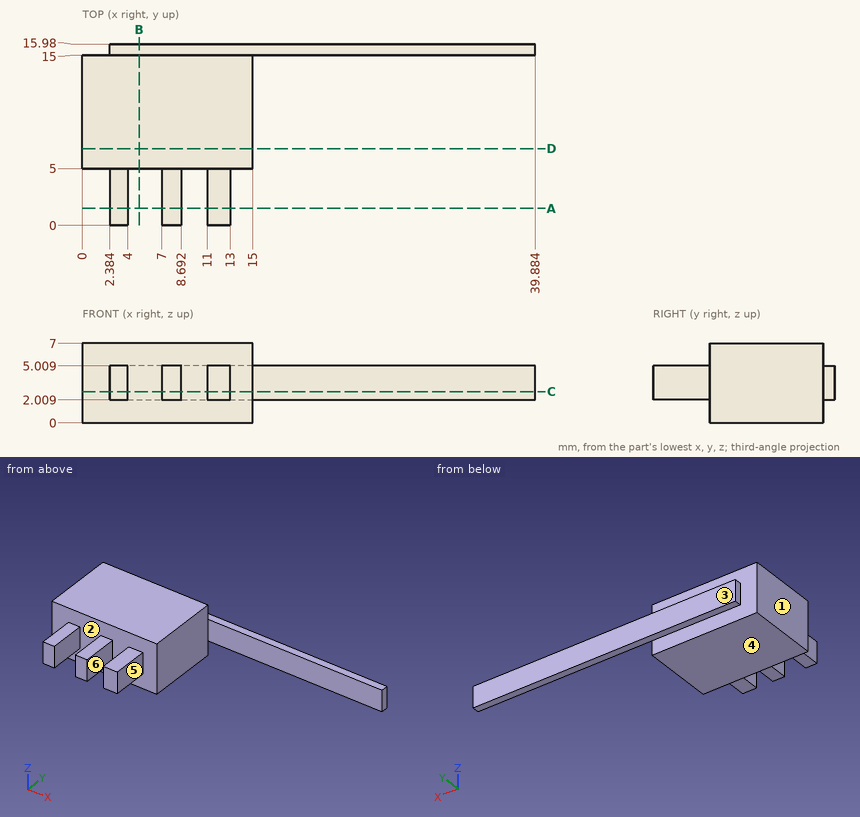
Print and shaded views of the part. All mm, measured from the part's lowest x, y and z. A direction names the side the tool comes from. Give positions to 0.01 mm unless a question says otherwise; leave off trailing zeros. Loops run counter-clockwise (first coordinate to the right, second up) from the corner with the lowest first, then second, coordinate; pieces in that order, holes last. Notation, with made-up numbers: (71.25, 87.5) - (89.25, 87.5) arc R15 cw to (89.25, 115.5) - close; hole circle Ø10 at (-26.5, 7.25). An arc over 180 degrees is marked (long way). One line per item, written item: value. Start each with the question number.
1. Slice it at B-B (x = 5). List the corners of the cut face in (y, z).
2. Pull direction X, two halves, no side cores. Call the marked faces 1, 2 and 3: pulls with the +X half, pulls with the -X half, needs draft (parallel to the pull), parting line crosses it, or undercut.
3. Slice it at A-A (y = 1.5). List the corners of the cut face in (x, z).
4. Slice it at C-C (z = 2.75). List the corners of the cut face in (x, y), plus the area to 3 significant figures.
5. Slice it at D-D (y = 6.75). List the corners of the cut face in (x, z), plus the area to 3 significant figures.
6. Probe L1, parallel to X at y = 12, z = 4.25; L2, parallel to Y at x = 10, z = 4; L3, parallel to Y at x = 14.5, z = 1.75. List the from-to ranges inside material, lowest first. Write a range as from..to.
7. Which spindle directions (+Z, -Z, +X, -X, +Y, -Y) get a long thin tool onto all of the face, cutting with end or side? Do the marked faces 4, 5 and 6. Say none if no direction does.
8. Pin check, flat tips, straight feed: pin 1 (2 mm diameter, centred on x = 12, y = 3, fed in from -Z); pin 2 (0.9 mm diameter, centred on y = 3, z = 3, fed in from +X); pin 3 (1.8 mm diameter, centred on x = 3, y = 2.5, fed in from +Z). Stop position of each tip, or through.
Solution:
1. outline: (5, 0) - (15, 0) - (15, 2.01) - (15.98, 2.01) - (15.98, 5.01) - (15, 5.01) - (15, 7) - (5, 7) - close
2. face 1: pulls with the -X half
2. face 2: undercut
2. face 3: needs draft
3. outline: (2.38, 2.01) - (4, 2.01) - (4, 5.01) - (2.38, 5.01) - close; (7, 2.01) - (8.69, 2.01) - (8.69, 5.01) - (7, 5.01) - close; (11, 2.01) - (13, 2.01) - (13, 5.01) - (11, 5.01) - close
4. outline: (0, 5) - (2.38, 5) - (2.38, 0) - (4, 0) - (4, 5) - (7, 5) - (7, 0) - (8.69, 0) - (8.69, 5) - (11, 5) - (11, 0) - (13, 0) - (13, 5) - (15, 5) - (15, 15) - (39.88, 15) - (39.88, 15.98) - (2.38, 15.98) - (2.38, 15) - (0, 15) - close
4. area: 213 mm^2
5. outline: (0, 0) - (15, 0) - (15, 7) - (0, 7) - close
5. area: 105 mm^2
6. L1: x = 0..15
6. L2: y = 5..15.98
6. L3: y = 5..15
7. face 4: -Z, +X, -X, +Y, -Y
7. face 5: +Z, -Z, +X, -Y
7. face 6: +Z, -Z, -Y
8. pin 1: stops at z = 2.01
8. pin 2: stops at x = 13
8. pin 3: stops at z = 5.01
